```python
from build123d import *

# Parameters (mm, degrees)
SKETCH2_R                = 10
BOSS_EXTRUDE1_DEPTH      = 40
BOSS_EXTRUDE1_DEPTH_BACK = 40
SKETCH1_R                = 25.4
SKETCH1_R_2              = 12.7
BOSS_EXTRUDE2_DEPTH      = 12.7
BOSS_EXTRUDE2_DEPTH_BACK = 12.7


with BuildPart() as part:
    # Sketch2 → Boss-Extrude1 (new body, two sides)
    with BuildSketch(Plane(origin=(0, 0, 0), x_dir=(0, 0, -1), z_dir=(1, 0, 0))) as boss_extrude1_sk:
        Circle(SKETCH2_R)
    extrude(amount=BOSS_EXTRUDE1_DEPTH)
    extrude(boss_extrude1_sk.sketch, amount=-BOSS_EXTRUDE1_DEPTH_BACK)

    # Sketch1 → Boss-Extrude2 (add, two sides)
    with BuildSketch(Plane(origin=(0, 0, 0), x_dir=(1, 0, 0), z_dir=(0, 1, 0))) as boss_extrude2_sk:
        Circle(SKETCH1_R)
        Circle(SKETCH1_R_2, mode=Mode.SUBTRACT)
    extrude(amount=BOSS_EXTRUDE2_DEPTH)
    extrude(boss_extrude2_sk.sketch, amount=-BOSS_EXTRUDE2_DEPTH_BACK)


solid = part.part
```
Can you work these out from the model? Positions are in its coordinate system, mm. A direction names the side the tool comes from. Round coordinates to 2 decimals unless told otherwise and drop trailing zeros. Loops run counter-clockwise (first coordinate to the right, second up) from the corner with the lowest first, then second, coordinate; pieces in that order, holes last. Notation, with made-up numbers: M 75.5,22 L 99.5,22 A20 cw 99.5,33 Z; hole C 72.5,58.25 d9. An arc over 180 degrees is marked long. Write item = value, one per line. Start each with the question number.
(1) If we mould it in two halves opening along Z, with no side actions, what happens to faces 3 (the face through (5, -12.7, -12)), 4 (the face through (-31.56, -9.76, 2.17)), 5 (the face through (0.169, -3.83, -9.237))? For each: released by +Z, released by -Z, zero draft, split by the parting line, or undercut.
(2) Suppose I cut it at D-D on y = 8.75. Write out the boundary of the cut face in (x, z), plus the area to 3 significant figures.
(3) I need wall thicknesses on line 1 along Z through (x, y) = (-1, -1.25); line 2 along Z through (x, y) = (0, 8.25); line 3 along X through (y, z) = (-8.75, 8). Which ranges of each line are inside material? Lowest first, please.
(4) Which directions (+Z, -Z, +X, -X, +Y, -Y) give clear straight access to the entire face, cutting with the end or side of a thin tool? Please do faces 1 (the face through (32, 0, 10)), 2 (the face through (40, 0, 0)).
(5) Suppose I cut it at A-A on x = 0. Write out the boundary of the cut face in (y, z), plus the area to 3 significant figures.
(6) I'm going to push flat-ended pins straight in: P1, Ø8, axis at x = -9.5, y = -2, coming from the +Z side; P2, Ø4, axis at x = -10, y = -6.5, coming from the -Z side; P3, Ø1, axis at y = 1, z = -16.5, coming from the -X side. Where does each tip first touch, or does it pass through?
(7) Suppose I cut it at C-C on z = 0. Write out the boundary of the cut face in (x, y), plus the area to 3 significant figures.
(8) Suppose I cut it at B-B on y = -5.75. Write out the boundary of the cut face in (x, z).
Answer block:
q1.face_3 = zero draft
q1.face_4 = split by the parting line
q1.face_5 = undercut
q2.outline = M -40,-4.84 L -24.93,-4.84 A25.4 ccw 24.93,-4.84 L 40,-4.84 L 40,4.84 L 24.93,4.84 A25.4 ccw -24.93,4.84 L -40,4.84 Z; hole M -11.74,-4.84 A12.7 ccw 11.74,-4.84 Z; hole M -11.74,4.84 L 11.74,4.84 A12.7 ccw Z
q2.area = 2,050 mm²
q3.line_1 = -25.38 to -12.66, -9.92 to 9.92, 12.66 to 25.38
q3.line_2 = -25.4 to -12.7, -5.65 to 5.65, 12.7 to 25.4
q3.line_3 = -24.11 to -9.86, 9.86 to 24.11
q4.face_1 = +X
q4.face_2 = +Z, -Z, +X, +Y, -Y
q5.outline = M -12.7,-25.4 L 12.7,-25.4 L 12.7,-12.7 L -12.7,-12.7 Z; M -12.7,12.7 L 12.7,12.7 L 12.7,25.4 L -12.7,25.4 Z; C 0,0 d20
q5.area = 959 mm²
q6.P1 = 24.8
q6.P2 = -24.11
q6.P3 = -19.73
q7.outline = M -40,-10 L -25.4,-10 L -25.4,-12.7 L -12.7,-12.7 L -12.7,-10 L 12.7,-10 L 12.7,-12.7 L 25.4,-12.7 L 25.4,-10 L 40,-10 L 40,10 L 25.4,10 L 25.4,12.7 L 12.7,12.7 L 12.7,10 L -12.7,10 L -12.7,12.7 L -25.4,12.7 L -25.4,10 L -40,10 Z
q7.area = 1,740 mm²
q8.outline = M -40,-8.18 L -24.05,-8.18 A25.4 ccw 24.05,-8.18 L 40,-8.18 L 40,8.18 L 24.05,8.18 A25.4 ccw -24.05,8.18 L -40,8.18 Z; hole M -9.71,-8.18 A12.7 ccw 9.71,-8.18 Z; hole M -9.71,8.18 L 9.71,8.18 A12.7 ccw Z
